Part print with two shaded views. Sizes in mm from the minimum x, y, z corner. Round coordinates to 2 decimals unless told otherwise and drop trailing zeros. Order: outer loops, then holes, each group sorted by start corner. A loop starts at its lowest first (then second) coordinate and runs counter-clockwise, first axis right, second up. Notation, with made-up numbers: M 47.5,56 L 53.5,56 A35 cw 53.5,89 Z; hole C 49,58 d11. An arc over 180 degrees is marked long. Answer as a JSON object with one key per item and string values.
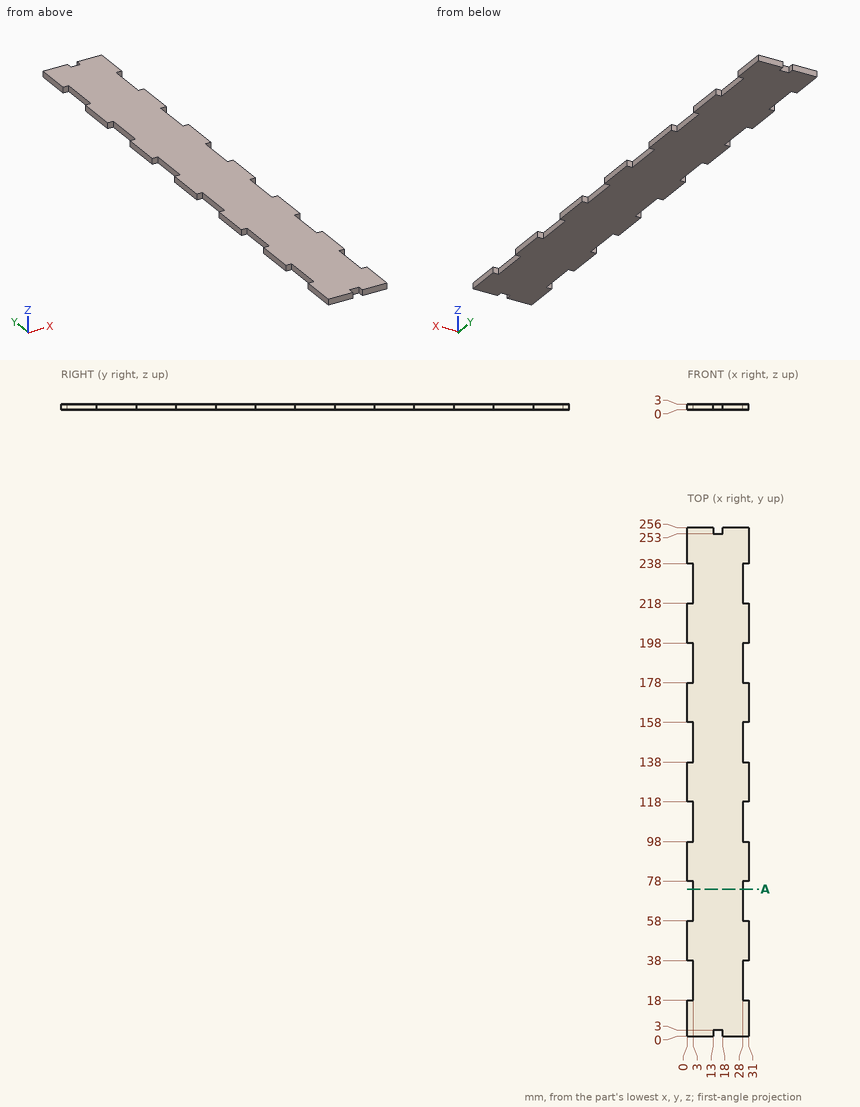
Item 1: Drop flat-ended pins along their axis: pin 1 Ø0.9 at (x, z) = (14.5, 2) entering from +Y; pin 2 Ø0.9 at (y, z) = (110.5, 2) entering from -X; pin 3 Ø1.5 at (y, z) = (26.5, 1.5) entering from +X. Give the stop position or say it passes through.
Worked answers:
{"pin 1": "stops at y = 253", "pin 2": "stops at x = 3", "pin 3": "stops at x = 28"}
Item 2: Saw through at A-A on y = 74. List the corners of the cut face in (x, z), and give its area (3 significant figures).
Worked answers:
{"outline": "M 3,0 L 28,0 L 28,3 L 3,3 Z", "area": "75.0 mm2"}
Item 3: Wall check: line 1 along X through (y, z) = (103.5, 0.2); line 2 along Y through (x, z) = (13.5, 0.6). Give the ranges that are in metal, low to high. Write a range as [from, to].
Worked answers:
{"line 1": "x = [3, 28]", "line 2": "y = [3, 253]"}
